Verification items for this drawing (mm, ordinates from the low corner). A direction names the side the tool comes from. Round coordinates to 2 decimals unless told otherwise and drop trailing zeros. Order: outer loops, then holes, each group sorted by start corner. A loop starts at its lowest first (then second) coordinate and runs counter-clockwise, first axis right, second up. Notation, with made-up numbers: (-23, 21.5) -> (33, 21.5) arc R20 cw to (33, 35.5) -> close; hole circle Ø1 at (12.5, 13). An arc over 180 degrees is marked (long way). Answer in a Markdown table with one row per item.
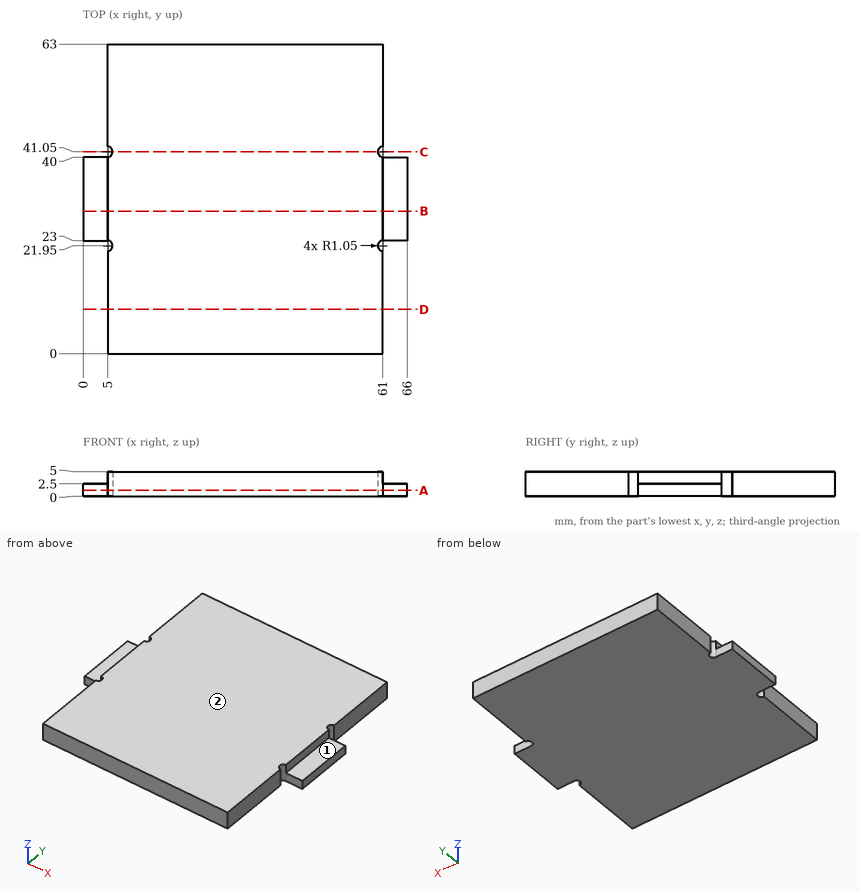
Item 1: Cross-section at D-D (y = 9). Record the boundary of the cut face in (x, z).
Result sheet:
| item | result |
|---|---|
| outline | (5, 0) -> (61, 0) -> (61, 5) -> (5, 5) -> close |
Item 2: Cross-section at C-C (y = 41.05). Record the boundary of the cut face in (x, z).
Result sheet:
| item | result |
|---|---|
| outline | (6.05, 0) -> (59.95, 0) -> (59.95, 5) -> (6.05, 5) -> close |
Item 3: Scan lines: line 1 (X direction, y = 9, z = 2); line 2 (X direction, y = 40.5, z = 3.6). Record each from-to range of solid material in increasing order. Write a range as [from, to].
Result sheet:
| item | result |
|---|---|
| line 1 | x = [5, 61] |
| line 2 | x = [5.89, 60.11] |
Item 4: Depth check by flat-ended pin: P1, Ø1.2, axis at y = 35, z = 4, coming from the +X side; P2, Ø2.5, axis at x = 1.5, y = 32, coming from the +Z side; P3, Ø2.5, axis at y = 56.5, z = 2.5, coming from the -X side. Enter the tip coordinate at first touch or a pass-through.
Result sheet:
| item | result |
|---|---|
| P1 | stops at x = 61 |
| P2 | stops at z = 2.5 |
| P3 | stops at x = 5 |
Item 5: Cross-section at A-A (z = 1.2). Record the boundary of the cut face in (x, y), and give its area (3 significant figures).
Result sheet:
| item | result |
|---|---|
| outline | (0, 23) -> (5, 23) arc R1.05 cw to (5, 20.9) -> (5, 0) -> (61, 0) -> (61, 20.9) arc R1.05 cw to (61, 23) -> (66, 23) -> (66, 40) -> (61, 40) arc R1.05 cw to (61, 42.1) -> (61, 63) -> (5, 63) -> (5, 42.1) arc R1.05 cw to (5, 40) -> (0, 40) -> close |
| area | 3,690 mm^2 |
Item 6: Set-up check for the marked faces 1 and 2: record each of +Z, -Z, +X, -X, +Y, -Y from which the full face is reachable in a straight line by a thin tool's end or side.
Result sheet:
| item | result |
|---|---|
| face 1 | +Z, +X, +Y, -Y |
| face 2 | +Z, +X, -X, +Y, -Y |
Item 7: Cross-section at B-B (y = 29). Record the boundary of the cut face in (x, z), and give its area (3 significant figures).
Result sheet:
| item | result |
|---|---|
| outline | (0, 0) -> (66, 0) -> (66, 2.5) -> (61, 2.5) -> (61, 5) -> (5, 5) -> (5, 2.5) -> (0, 2.5) -> close |
| area | 305 mm^2 |
